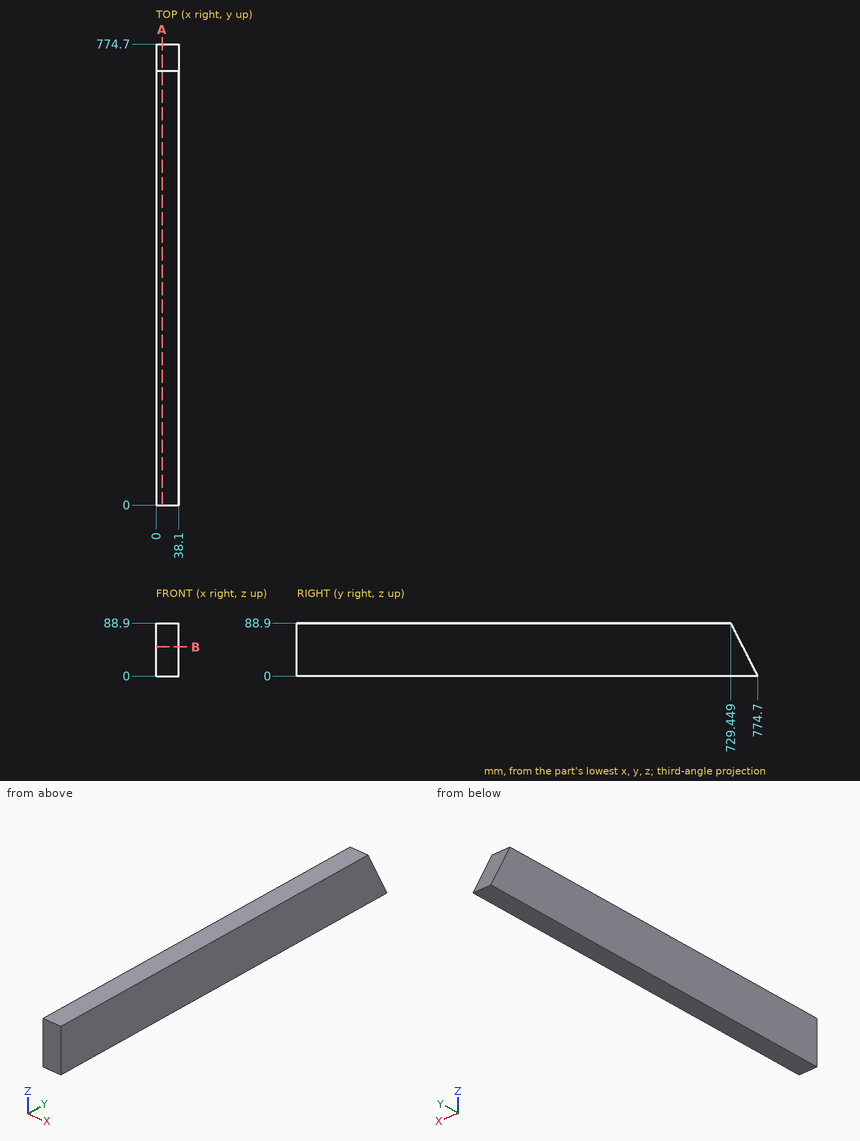
Study the drawing (mm; zero at the part's minimum x, y, z) and answer. Round coordinates to 2 decimals unless told otherwise and drop trailing zeros. Write each loop counter-clockwise with the first axis right and the second up, starting at its lowest first coordinate (ties: lowest second). Pieces come first, ordered by that corner, then holes. Notation, with made-up numbers: (47.5, -3.5) -> (91.5, -3.5) arc R29 ccw to (91.5, 27.5) -> close; hole circle Ø10 at (-31, -11.5). An arc over 180 degrees is marked (long way). Use CSV: the item, a comma, the result in double quotes. Start each with the question number.
(1) Consider L1, parallel to Y at x = 6, z = 62.5 (1 decimal); L2, parallel to Y at x = 8, z = 58.5. Determine where each line is inside the solid, lowest interval first. Write a range as from..to.
(2) Section A-A on x = 10 is taken. Give the vertices of the cut face in (y, z), then the cut area to 3 significant figures.
(3) Section B-B on z = 49 is taken. Give the vertices of the cut face in (x, y).
A:
1,L1,"y = 0..742.9"
1,L2,"y = 0..744.92"
2,outline,"(0, 0) -> (774.7, 0) -> (729.45, 88.9) -> (0, 88.9) -> close"
2,area,"66,900 mm²"
3,outline,"(0, 0) -> (38.1, 0) -> (38.1, 749.76) -> (0, 749.76) -> close"
